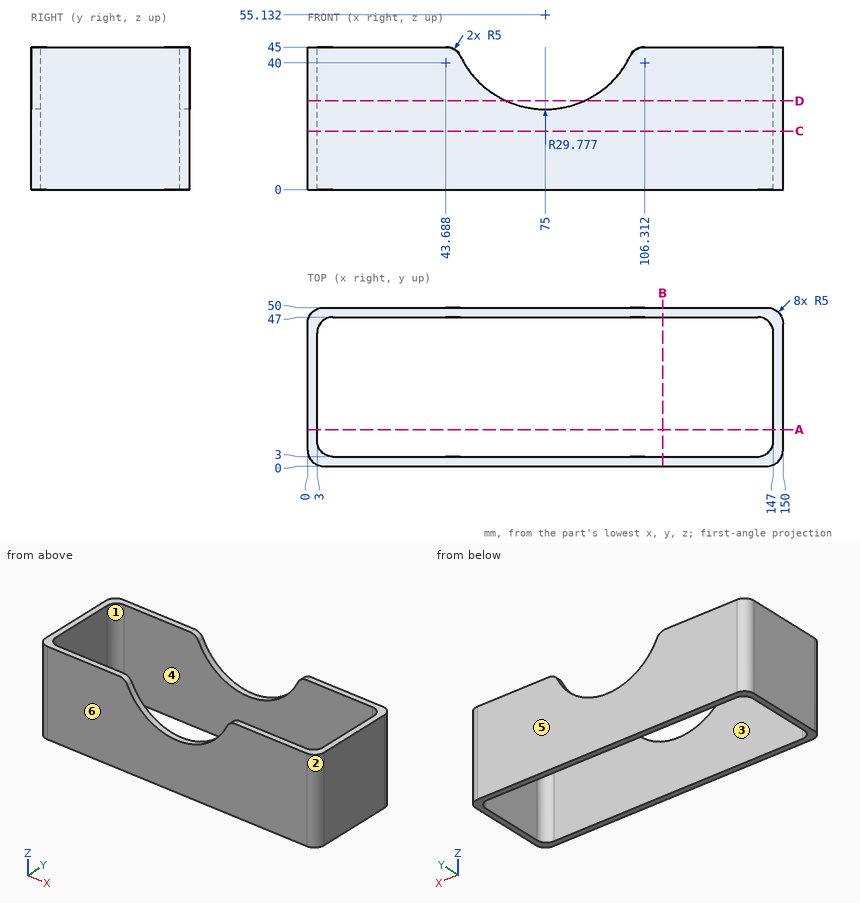
Print and shaded views of the part. All mm, measured from the part's lowest x, y and z. A direction names the side the tool comes from. Coordinates: 2 decimals unless noted, no trailing zeros. Loops run counter-clockwise (first coordinate to the right, second up) from the corner with the lowest first, then second, coordinate; pieces in that order, holes last. Notation, with made-up numbers: (56.25, 62) - (110.25, 62) arc R13 ccw to (110.25, 78) - close; hole circle Ø5 at (67.25, 71). An arc over 180 degrees is marked (long way). Use one line per item in the form item = value. Start each with the question number.
1) Band-saw the part on C-C (z = 18.5). Give the cut face in (x, y), and give its area (3 significant figures).
2) Two-plate mould, pull along Y, no slides. Class the marked faces 3, 4, 5 and 6: +Y half, -Y half, draft (parallel to the pull), parting line (faces both ways), or undercut.
3) Drill centre lines: L1, parallel to X at y = 12.5, z = 6; L2, parallel to Y at x = 125, z = 15; L3, parallel to X at y = 5, z = 10.5. Where is each one in solid material? Low to high. Write a range as from..to.
4) Band-saw the part on A-A (y = 11.5). Give the cut face in (x, z).
5) Band-saw the part on D-D (z = 28). Give the cut face in (x, y).
6) Band-saw the part on B-B (x = 112). Give the cut face in (y, z).
7) Tool access for the marked faces 1 and 2: list every direction of +Z, -Z, +X, -X, +Y, -Y with a clear straight run to the whole face (end or side of a thin tool).
Check values:
q1.outline = (0, 5) arc R5 ccw to (5, 0) - (145, 0) arc R5 ccw to (150, 5) - (150, 45) arc R5 ccw to (145, 50) - (5, 50) arc R5 ccw to (0, 45) - close; hole (3, 8) arc R5 ccw to (8, 3) - (142, 3) arc R5 ccw to (147, 8) - (147, 42) arc R5 ccw to (142, 47) - (8, 47) arc R5 ccw to (3, 42) - close
q1.area = 1,160 mm2
q2.face_3 = undercut
q2.face_4 = undercut
q2.face_5 = +Y half
q2.face_6 = -Y half
q3.L1 = 0..3, 147..150
q3.L2 = 0..3, 47..50
q3.L3 = 0..4, 146..150
q4.outline = (0, 0) - (3, 0) - (3, 45) - (0, 45) - close; (147, 0) - (150, 0) - (150, 45) - (147, 45) - close
q5.outline = (0, 5) arc R5 ccw to (5, 0) - (62.73, 0) - (62.73, 3) - (8, 3) arc R5 cw to (3, 8) - (3, 42) arc R5 cw to (8, 47) - (62.73, 47) - (62.73, 50) - (5, 50) arc R5 ccw to (0, 45) - close; (87.27, 0) - (145, 0) arc R5 ccw to (150, 5) - (150, 45) arc R5 ccw to (145, 50) - (87.27, 50) - (87.27, 47) - (142, 47) arc R5 cw to (147, 42) - (147, 8) arc R5 cw to (142, 3) - (87.27, 3) - close
q6.outline = (0, 0) - (3, 0) - (3, 45) - (0, 45) - close; (47, 0) - (50, 0) - (50, 45) - (47, 45) - close
q7.face_1 = +Z, -Z
q7.face_2 = +Z, -Z, +X, -Y
